Design review of the part built by this model. Coordinates are the model's own, in mm. Coordinates: 2 decimals unless noted, no trailing zeros. Loops run counter-clockwise (first coordinate to the right, second up) from the corner with the lowest first, then second, coordinate; pieces in that order, holes last. Notation, with made-up numbers: (-33.5, -15) -> (15.5, -15) arc R22 ccw to (15.5, 16) -> close; hole circle Ø11 at (21.25, -39). An arc over 180 degrees is marked (long way). Answer as a JSON object with one key per item and string values.
```python
from build123d import *

# Parameters (mm, degrees)
PAD_DEPTH = 1000


with BuildPart() as part:
    # Sketch → Pad (new body)
    with BuildSketch(Plane.XZ):
        with BuildLine():
            Line((0, 0), (5, 0))
            Line((5, 0), (5, 13))
            Line((5, 13), (0.288833, 29.781088))
            ThreePointArc((0.288833, 29.781088), (0.181209, 29.939088), (0, 30))
            Line((0, 22.336099), (0, 30))
            ThreePointArc((0.481389, 21.971245), (0.302016, 22.234579), (0, 22.336099))
            Line((0.481389, 21.971245), (3, 13))
            Line((3, 13), (3, 2))
            Line((3, 2), (0, 2))
            Line((0, 2), (0, 0))
        make_face()
    pad = extrude(amount=-PAD_DEPTH)

    # Mirrored: Pad across Sketch V_Axis
    add(pad.mirror(Plane(origin=(0, 0, 0), x_dir=(0, -1, 0), z_dir=(1, 0, 0))))


solid = part.part
```
1) Wall thickness on probe 1 along X at (y, z) = (945, 4.75); probe 2 along Z at (x, y) = (0, 656); probe 3 along Z at (x, y) = (0.25, 490): over which ranges is each line inside the solid? List them lowest first.
Completed:
{"probe 1": "-5 to -3, 3 to 5", "probe 2": "0 to 2, 22.34 to 30", "probe 3": "0 to 2, 22.27 to 29.87"}
2) Clearance check with flat-ended pins moving along their axes: pin 1 Ø2 at (y, z) = (639.5, 20) entering from +X; pin 2 Ø5 at (y, z) = (666, 25) entering from +X; pin 3 Ø6 at (y, z) = (274.5, 24) entering from +X. State where each tip first meets the part, or that it passes through.
Completed:
{"pin 1": "x = 3.32", "pin 2": "x = 2.33", "pin 3": "x = 2.75"}
3) Add section A-A, the plane y = 599.5. Give the boundary of the cut face in (x, z).
Completed:
{"outline": "(-5, 0) -> (5, 0) -> (5, 13) -> (0.29, 29.78) arc R0.3 ccw to (0, 30) arc R0.3 ccw to (-0.29, 29.78) -> (-5, 13) -> close; hole (-3, 2) -> (3, 2) -> (3, 13) -> (0.48, 21.97) arc R0.5 ccw to (-0.48, 21.97) -> (-3, 13) -> close"}
